```python
from build123d import *

# Parameters (mm, degrees)
SKETCH2_W           = 40
SKETCH2_H           = 40
BOSS_EXTRUDE1_DEPTH = 30
SKETCH6_W           = 26
SKETCH6_H           = 26
BOSS_EXTRUDE2_DEPTH = 40
SKETCH7_R           = 11
CUT_EXTRUDE3_DEPTH  = 7
SKETCH3_R           = 6
CUT_EXTRUDE4_DEPTH  = 5
SKETCH4_R           = 10
CUT_EXTRUDE5_DEPTH  = 25


with BuildPart() as part:
    # Sketch2 → Boss-Extrude1 (new body)
    with BuildSketch(Plane.XY):
        Rectangle(SKETCH2_W, SKETCH2_H)
    extrude(amount=BOSS_EXTRUDE1_DEPTH)

    # Sketch6 → Boss-Extrude2 (add)
    with BuildSketch(Plane(origin=(20, 0, 0), x_dir=(0, 0, -1), z_dir=(1, 0, 0))):
        with Locations((-15, 0)):
            Rectangle(SKETCH6_W, SKETCH6_H)
    extrude(amount=-BOSS_EXTRUDE2_DEPTH)

    # Sketch7 → Cut-Extrude3 (cut)
    with BuildSketch(Plane(origin=(20, 0, 0), x_dir=(0, 0, -1), z_dir=(1, 0, 0))):
        with Locations((-15, 0)):
            Circle(SKETCH7_R)
    extrude(amount=-CUT_EXTRUDE3_DEPTH, mode=Mode.SUBTRACT)

    # Sketch3 → Cut-Extrude4 (cut)
    with BuildSketch(Plane.XY.offset(30)):
        Circle(SKETCH3_R)
    extrude(amount=-CUT_EXTRUDE4_DEPTH, mode=Mode.SUBTRACT)

    # Sketch4 → Cut-Extrude5 (cut)
    with BuildSketch(Plane(origin=(0, 0, 0), x_dir=(-1, 0, 0), z_dir=(0, 0, -1))):
        Circle(SKETCH4_R)
    extrude(amount=-CUT_EXTRUDE5_DEPTH, mode=Mode.SUBTRACT)


solid = part.part
```
Read the model definition and answer for the solid it produces. Units are mm, in the model's axes. A direction names the side the tool comes from. Round coordinates to 2 decimals unless told otherwise and drop trailing zeros. Write each loop counter-clockwise with the first axis right and the second up, starting at its lowest first coordinate (ties: lowest second). Pieces come first, ordered by that corner, then holes. Notation, with made-up numbers: M 77.5,80.5 L 124.5,80.5 A34 cw 124.5,117.5 Z; hole C -39.5,-2 d2. An arc over 180 degrees is marked long. One line per item, written item: value.
Q1. Find section C-C on z = 15. Write down the section's boundary in (x, y).
Data:
outline: M -20,-20 L 20,-20 L 20,-11 L 13,-11 L 13,11 L 20,11 L 20,20 L -20,20 Z; hole C 0,0 d20
Q2. For a pull along X with two mould halves and no side action, classify faces 4 (the cylindrical face through (-6, 0, 28)), 5 (the flat face through (20, -5, 5)), 6 (the flat face through (0, -20, 15)) as +X half, -X half, draft (parallel to the pull), parting line (faces both ways), or undercut.
Data:
face 4: undercut
face 5: +X half
face 6: draft
Q3. Flat-ended cylindrical pins translate along their axes: pin 1 Ø5 at (y, z) = (3, 17) entering from +X; pin 2 Ø22 at (x, y) = (-4.5, 0) entering from -Z. Find the tip coordinate at first contact, or state that the pin passes through.
Data:
pin 1: x = 13
pin 2: z = 0
Q4. Find section B-B on x = 0. Write down the section's boundary in (y, z), plus the area to 3 significant figures.
Data:
outline: M -20,0 L -10,0 L -10,25 L -6,25 L -6,30 L -20,30 Z; M 6,25 L 10,25 L 10,0 L 20,0 L 20,30 L 6,30 Z
area: 640 mm2
Q5. Find section A-A on y = 0. Write down the section's boundary in (x, z), plus the area to 3 significant figures.
Data:
outline: M -20,0 L -10,0 L -10,25 L -6,25 L -6,30 L -20,30 Z; M 6,25 L 10,25 L 10,0 L 20,0 L 20,4 L 13,4 L 13,26 L 20,26 L 20,30 L 6,30 Z
area: 486 mm2
Q6. Find section D-D on x = 16. Write down the section's boundary in (y, z), plus the area to 3 significant figures.
Data:
outline: M -20,0 L 20,0 L 20,30 L -20,30 Z; hole C 0,15 d22
area: 820 mm2
Q7. Which of the six approach directions +Z, -Z, +X, -X, +Y, -Y give full straight-line access (tool end or side, diameter ignored) to faces 1 (the flat face through (0, 20, 15)), 2 (the cylindrical face through (2.17, -9.76, 12.32)), 3 (the cylindrical face through (16.549, -4.213, 4.839))?
Data:
face 1: +Z, -Z, +X, -X, +Y
face 2: -Z
face 3: +X
Q8. Straight lines are drawn through the part: line 1 (Y direction, x = 0, z = 11.75); line 2 (Y direction, x = 17, z = 15); line 3 (X direction, y = -7.5, z = 3.5). For each, find the intervals that lie inside material, in ascending order. Write a range as [from, to].
Data:
line 1: [-20, -10], [10, 20]
line 2: [-20, -11], [11, 20]
line 3: [-20, -6.61], [6.61, 20]
